from build123d import *

# Parameters (mm, degrees)
F0_R      = 19.685
F0_R_2    = 10.16
F0_R_3    = 8.89
F1_DEPTH  = 24.892
F2_R      = 19.685
F2_R_2    = 3.175
F3_DEPTH  = 8.382
F4_R      = 9.271
F5_DEPTH  = 8.89
F6_R      = 9.271
F6_R_2    = 3.175
F7_DEPTH  = 5.08
F8_R      = 3.81
F8_R_2    = 3.175
F9_DEPTH  = 2.54
F10_R     = 1.778
F11_DEPTH = 7.6708
F12_R     = 0.1524
F13_DEPTH = 0.3175
F15_R     = 17.78
F15_R_2   = 10.16
F16_DEPTH = 12.7


with BuildPart() as f1:
    # F0 (on Front) → F1 (new body)
    with BuildSketch(Plane.XZ):
        Circle(F0_R)
        Circle(F0_R_2, mode=Mode.SUBTRACT)
        Circle(F0_R_2)
        Circle(F0_R_3, mode=Mode.SUBTRACT)
        Circle(F0_R_3)
    extrude(amount=F1_DEPTH)

    # F2 (on face) → F3 (cut)
    with BuildSketch(Plane(origin=(0, 0, 0), x_dir=(-1, 0, 0), z_dir=(0, 1, 0))):
        Circle(F2_R)
        Circle(F2_R_2, mode=Mode.SUBTRACT)
    extrude(amount=-F3_DEPTH, mode=Mode.SUBTRACT)

    # F4 (on face) → F5 (cut)
    with BuildSketch(Plane.XZ.offset(24.892)):
        Circle(F4_R)
    extrude(amount=-F5_DEPTH, mode=Mode.SUBTRACT)

    # F6 (on face) → F7 (cut)
    with BuildSketch(Plane.XZ.offset(16.002)):
        Circle(F6_R)
        Circle(F6_R_2, mode=Mode.SUBTRACT)
    extrude(amount=-F7_DEPTH, mode=Mode.SUBTRACT)

    # F8 (on face) → F9 (join)
    with BuildSketch(Plane.XZ.offset(10.922)):
        Circle(F8_R)
        Circle(F8_R_2, mode=Mode.SUBTRACT)
    extrude(amount=F9_DEPTH)

    # F10 (on face) → F11 (cut)
    with BuildSketch(Plane.XZ.offset(10.922)):
        with Locations((-4.6248319024, 4.6248319024)):
            Circle(F10_R)
        with BuildLine():
            ThreePointArc((1.778, 6.5405), (-1.2572358569, 7.7977358569), (0, 4.7625))
            ThreePointArc((0, 4.7625), (1.2572358569, 5.2832641431), (1.778, 6.5405))
        make_face()
        with Locations((4.6248319024, 4.6248319024)):
            Circle(F10_R)
        with Locations((6.5405, 0)):
            Circle(F10_R)
        with Locations((4.6248319024, -4.6248319024)):
            Circle(F10_R)
        with Locations((0, -6.5405)):
            Circle(F10_R)
        with Locations((-4.6248319024, -4.6248319024)):
            Circle(F10_R)
        with Locations((-6.5405, 0)):
            Circle(F10_R)
    extrude(amount=-F11_DEPTH, mode=Mode.SUBTRACT)

    # F12 (on face) → F13 (join)
    with BuildSketch(Plane.XZ.offset(13.462)):
        with BuildLine():
            ThreePointArc((0.1524, 3.4925), (-0.1077630735, 3.6002630735), (0, 3.3401))
            ThreePointArc((0, 3.3401), (0.1077630735, 3.3847369265), (0.1524, 3.4925))
        make_face()
        with Locations((2.0528399936, 2.8254918529)):
            Circle(F12_R)
        with Locations((3.3215648832, 1.0792418529)):
            Circle(F12_R)
        with Locations((3.3215648832, -1.0792418529)):
            Circle(F12_R)
        with Locations((2.0528399936, -2.8254918529)):
            Circle(F12_R)
        with Locations((0, -3.4925)):
            Circle(F12_R)
        with Locations((-2.0528399936, -2.8254918529)):
            Circle(F12_R)
        with Locations((-3.3215648832, -1.0792418529)):
            Circle(F12_R)
        with Locations((-3.3215648832, 1.0792418529)):
            Circle(F12_R)
        with Locations((-2.0528399936, 2.8254918529)):
            Circle(F12_R)
    extrude(amount=F13_DEPTH)

    # F15 (on face) → F16 (cut)
    with BuildSketch(Plane(origin=(0, -8.382, 0), x_dir=(-1, 0, 0), z_dir=(0, 1, 0))):
        Circle(F15_R)
        Circle(F15_R_2, mode=Mode.SUBTRACT)
    extrude(amount=-F16_DEPTH, mode=Mode.SUBTRACT)


solid = f1.part
Verification items for the finished model (mm, model axes). A direction names the side the tool comes from. Round coordinates to 2 decimals unless told otherwise and drop trailing zeros. Loops run counter-clockwise (first coordinate to the right, second up) from the corner with the lowest first, then second, coordinate; pieces in that order, holes last. Notation, with made-up numbers: (18, 5.25) - (68, 5.25) arc R30 ccw to (68, 33.25) - close; hole circle Ø4 at (67.25, 82.25). An arc over 180 degrees is marked (long way). Use a Markdown table: item, result. Add a question column.
1. Section check C-C, the plane z = 16.5. Record the boundary of the cut face in (x, y).
2. Section check B-B, the plane y = -14.5. Record the boundary of the cut face in (x, z) (3 decimals), plus the area to 3 significant figures.
3. Access from +Z, -Z, +X, -X, +Y, -Y to the whole of each face (thin tool, end or side, straight path). Record for faces 1 (the face through (3.85, -14.64, -17.36)), 2 (the face through (-0.83, -12.17, -3.72)), 3 (the face through (-0.385, -9.67, -8.276)).
4. Release check for a two-part mould opening along Z. For faces 4 (the face through (0.69, -4.13, -3.1)), 5 (the face through (0, -16.002, 0)), 6 (the face through (4.1, -24.892, -8.5)), 7 (the face through (4.2, -9.7, 2.9)) record: released by +Z, released by -Z, zero draft, split by the parting line, or undercut.
5. Thickness scan on probe 1 along Z at (x, y) = (0, -9.15) (1 decimal); probe 2 along Z at (x, y) = (0, -20.5) (3 decimals); probe 3 along Z at (x, y) = (0, -11.5) (3 decimals). Record the ranges inside material, lowest first. Write a range as [from, to].
6. Section check A-A, the plane y = -9. Give the number of separate pieces and of enclosed holes in the cut face, plus the area to 3 significant figures.
7. Section check D-D, the plane y = -19. Record the boundary of the cut face in (x, z) (3 decimals).
8. Gauge pin test, flat ends, axial feed: pin 1 (4 mm diameter, centred on x = -6.54, z = 0, fed in from +Y); pin 2 (10 mm diameter, centred on x = 4, y = -16.5, fed in from -Z) (3 decimals); pin 3 (12 mm diameter, centred on x = 12, y = -3.5, fed in from -Z); pin 4 (2 mm diameter, centred on x = 0, z = -6.54, fed in from -Y). Record the tip position at first contact, or that the pin passes through.
Checks:
| question | item | result |
|---|---|---|
| 1 | outline | (-10.74, -24.89) - (10.74, -24.89) - (10.74, -8.38) - (6.62, -8.38) - (6.62, -21.08) - (-6.62, -21.08) - (-6.62, -8.38) - (-10.74, -8.38) - close |
| 2 | outline | circle Ø39.37 at (0, 0); circle Ø20.32 at (0, 0); circle Ø6.35 at (0, 0); hole circle Ø35.56 at (0, 0); hole circle Ø18.542 at (0, 0) |
| 2 | area | 310 mm^2 |
| 3 | face 1 | +Y |
| 3 | face 2 | -Y |
| 3 | face 3 | +Y, -Y |
| 4 | face 4 | split by the parting line |
| 4 | face 5 | undercut |
| 4 | face 6 | zero draft |
| 4 | face 7 | undercut |
| 5 | probe 1 | z = [-19.7, -17.8], [-10.2, -8.3], [-4.8, 4.8], [8.3, 10.2], [17.8, 19.7] |
| 5 | probe 2 | z = [-19.685, -17.78], [-10.16, -9.271], [9.271, 10.16], [17.78, 19.685] |
| 5 | probe 3 | z = [-19.685, -17.78], [-10.16, -9.271], [-3.81, 3.81], [9.271, 10.16], [17.78, 19.685] |
| 6 | separate pieces | 2 |
| 6 | enclosed holes | 9 |
| 6 | area | 469 mm^2 |
| 7 | outline | circle Ø39.37 at (0, 0); circle Ø20.32 at (0, 0); hole circle Ø35.56 at (0, 0); hole circle Ø18.542 at (0, 0) |
| 8 | pin 1 | stops at y = -8.38 |
| 8 | pin 2 | stops at z = -19.685 |
| 8 | pin 3 | stops at z = -17.75 |
| 8 | pin 4 | passes through |
